from build123d import *

# Parameters (mm, degrees)
SKETCH1_W              = 19.05
SKETCH1_H              = 76.2
BOSS_EXTRUDE1_DEPTH    = 2.54
SKETCH2_R              = 5.715
SKETCH2_R_2            = 3.175
BOSS_EXTRUDE2_DEPTH    = 76.2
SKETCH3_W              = 25.4
SKETCH3_H              = 6.35
SKETCH3_H_2            = 12.7
CUT_EXTRUDE1_DEPTH     = 80.372459959
F_10_CLEARANCE_HOLE1_D = 5.1054


with BuildPart() as part:
    # Sketch1 → Boss-Extrude1 (new body)
    with BuildSketch(Plane.XY):
        with Locations((-9.525, 38.1)):
            Rectangle(SKETCH1_W, SKETCH1_H)
    extrude(amount=BOSS_EXTRUDE1_DEPTH)

    # Sketch2 → Boss-Extrude2 (add)
    with BuildSketch(Plane(origin=(0, 0, 0), x_dir=(-1, 0, 0), z_dir=(0, -1, 0))):
        with Locations((0, -5.715)):
            Circle(SKETCH2_R)
        with Locations(Location((0, -5.715, 0), (0, 0, 90))):
            Circle(SKETCH2_R_2, mode=Mode.SUBTRACT)
    extrude(amount=-BOSS_EXTRUDE2_DEPTH)

    # Sketch3 → Cut-Extrude1 (cut, through all)
    with BuildSketch(Plane(origin=(0, 0, 0), x_dir=(-1, 0, 0), z_dir=(0, 0, -1))):
        with Locations((-2.54, 3.175)):
            Rectangle(SKETCH3_W, SKETCH3_H)
        with Locations((-2.54, 73.025)):
            Rectangle(SKETCH3_W, SKETCH3_H)
        with Locations((-2.54, 38.1)):
            Rectangle(SKETCH3_W, SKETCH3_H_2)
    extrude(amount=-CUT_EXTRUDE1_DEPTH, mode=Mode.SUBTRACT)

    # #10 Clearance Hole1 (through all)
    with Locations(Plane.XY.offset(2.54)):
        with Locations((-13.97, 63.5), (-13.97, 12.7)):
            Hole(F_10_CLEARANCE_HOLE1_D / 2)


solid = part.part
Build history of the part. All positions in model axes, mm. A direction names the side the tool comes from. Give positions to 0.01 mm unless a question says otherwise; leave off trailing zeros. Loops run counter-clockwise (first coordinate to the right, second up) from the corner with the lowest first, then second, coordinate; pieces in that order, holes last. Notation, with made-up numbers: (-3, -20.5) -> (16, -20.5) arc R21 ccw to (16, -5.5) -> close; hole circle Ø2 at (33, 55.25). An arc over 180 degrees is marked (long way). Answer in a Markdown table with one row per item.
Item 1: Slice it at B-B on x = -13.97. Write the cut outline in (y, z).
Findings below:
| item | result |
|---|---|
| outline | (0, 0) -> (10.15, 0) -> (10.15, 2.54) -> (0, 2.54) -> close; (15.25, 0) -> (60.95, 0) -> (60.95, 2.54) -> (15.25, 2.54) -> close; (66.05, 0) -> (76.2, 0) -> (76.2, 2.54) -> (66.05, 2.54) -> close |
Item 2: Flat gauge pins, fed straight in: P1, Ø5.5, axis at x = -2, z = 3.5, coming from the +Y side; P2, Ø2, axis at y = 74.5, z = 1, coming from the +X side; P3, Ø4.5, axis at x = -11, y = 33, coming from the +Z side. Where does each tip first touch, or does it go through?
Findings below:
| item | result |
|---|---|
| P1 | stops at y = 69.85 |
| P2 | stops at x = -10.16 |
| P3 | stops at z = 2.54 |
Item 3: Slice it at C-C on z = 3.5. Write the cut outline in (x, y).
Findings below:
| item | result |
|---|---|
| outline | (-5.27, 6.35) -> (-2.27, 6.35) -> (-2.27, 31.75) -> (-5.27, 31.75) -> close; (-5.27, 44.45) -> (-2.27, 44.45) -> (-2.27, 69.85) -> (-5.27, 69.85) -> close; (2.27, 6.35) -> (5.27, 6.35) -> (5.27, 31.75) -> (2.27, 31.75) -> close; (2.27, 44.45) -> (5.27, 44.45) -> (5.27, 69.85) -> (2.27, 69.85) -> close |
Item 4: Probe line 1 along Y through (x, z) = (-13.97, 1.9); line 2 along X through (y, z) = (31.5, 5.5); line 3 along Y through (x, z) = (-5.5, 1.75). List the from-to ranges inside material, lowest first. Write a range as [from, to].
Findings below:
| item | result |
|---|---|
| line 1 | y = [0, 10.15], [15.25, 60.95], [66.05, 76.2] |
| line 2 | x = [-5.71, -3.17], [3.17, 5.71] |
| line 3 | y = [6.35, 31.75], [44.45, 69.85] |
Item 5: Slice it at A-A on y = 63.5. Write the cut outline in (x, z) (3 decimals), plus the area to 3 significant figures.
Findings below:
| item | result |
|---|---|
| outline | (-19.05, 0) -> (-16.523, 0) -> (-16.523, 2.54) -> (-19.05, 2.54) -> close; (-11.417, 0) -> (0, 0) arc R5.715 ccw (long way) to (-4.752, 2.54) -> (-11.417, 2.54) -> close; hole circle Ø6.35 at (0, 5.715) |
| area | 97.9 mm² |
Item 6: Mould opens along Z. For faces 1 (the flat face through (-12, 39, 0)), 2 (the flat face through (-2, 6.35, 3)), 3 (the cylindrical face through (-1.932, 56.972, 8.235)) say: pulls with the +Z half, pulls with the -Z half, needs draft (parallel to the pull), parting line crosses it, or undercut.
Findings below:
| item | result |
|---|---|
| face 1 | pulls with the -Z half |
| face 2 | needs draft |
| face 3 | undercut |
Item 7: Tool access for faces 4 (the flat face through (-10.16, 38, 1)), 5 (the flat face through (-10.16, 73, 1)), 6 (the flat face through (-10.16, 3, 1)): list every direction of +Z, -Z, +X, -X, +Y, -Y with a clear straight run to the whole face (end or side of a thin tool).
Findings below:
| item | result |
|---|---|
| face 4 | +Z, -Z, +X |
| face 5 | +Z, -Z, +X, +Y |
| face 6 | +Z, -Z, +X, -Y |
Item 8: Slice it at D-D on x = 2.25. Write the cut outline in (y, z), plus the area to 3 significant figures.
Findings below:
| item | result |
|---|---|
| outline | (6.35, 0.46) -> (31.75, 0.46) -> (31.75, 3.47) -> (6.35, 3.47) -> close; (6.35, 7.96) -> (31.75, 7.96) -> (31.75, 10.97) -> (6.35, 10.97) -> close; (44.45, 0.46) -> (69.85, 0.46) -> (69.85, 3.47) -> (44.45, 3.47) -> close; (44.45, 7.96) -> (69.85, 7.96) -> (69.85, 10.97) -> (44.45, 10.97) -> close |
| area | 306 mm² |
